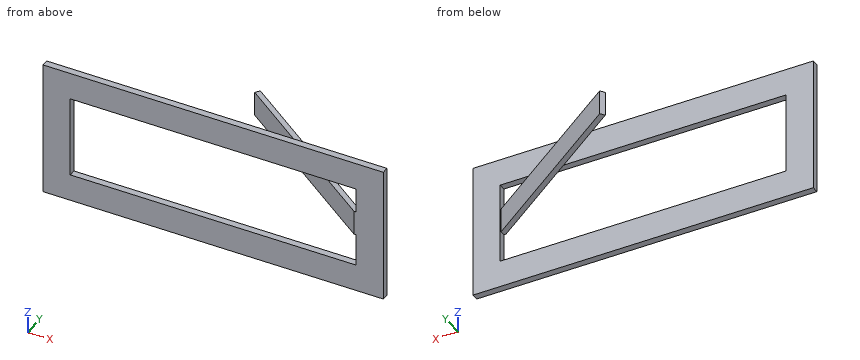
```python
from build123d import *

# Parameters (mm, degrees)
SKETCH1_W           = 20
SKETCH1_H           = 60
BOSS_EXTRUDE2_DEPTH = 10
BOSS_EXTRUDE3_DEPTH = 36
SKETCH3_W           = 140
SKETCH3_H           = 140
CUT_EXTRUDE1_DEPTH  = 18
SKETCH4_W           = 8.585490735
SKETCH4_H           = 18
CUT_EXTRUDE3_DEPTH  = 46
SKETCH5_W           = 250
SKETCH5_H           = 5
CUT_EXTRUDE4_DEPTH  = 137


with BuildPart() as part:
    # Sketch1 → Boss-Extrude2 (new body)
    with BuildSketch(Plane(origin=(0, 0, 0), x_dir=(1, 0, 0), z_dir=(0, 1, 0))):
        Polygon((166.222222222, 60), (146.222222222, 60), (-63.777777778, 60), (-83.777777778, 60), (-83.777777778, 80), (166.222222222, 80), align=None)
        with Locations((156.222222222, 30)):
            Rectangle(SKETCH1_W, SKETCH1_H)
        Polygon((166.222222222, 0), (146.222222222, 0), (-63.777777778, 0), (-83.777777778, 0), (-83.777777778, -20), (166.222222222, -20), align=None)
        with Locations((-73.777777778, 30)):
            Rectangle(SKETCH1_W, SKETCH1_H)
    extrude(amount=BOSS_EXTRUDE2_DEPTH)

    # Sketch2 → Boss-Extrude3 (add)
    with BuildSketch(Plane.XY):
        Polygon((155.307951765, 2.266232377), (27.198414629, 93.999150061), (24.869662654, 90.746933242), (148.437318839, 2.266232377), align=None)
    extrude(amount=-BOSS_EXTRUDE3_DEPTH)

    # Sketch3 → Cut-Extrude1 (cut)
    with BuildSketch(Plane.XY):
        with Locations((82.194738609, 80)):
            Rectangle(SKETCH3_W, SKETCH3_H)
    extrude(amount=-CUT_EXTRUDE1_DEPTH, mode=Mode.SUBTRACT)

    # Sketch4 → Cut-Extrude3 (cut)
    with BuildSketch(Plane(origin=(0, 10, 0), x_dir=(1, 0, 0), z_dir=(0, 1, 0))):
        with Locations((141.929476855, 9)):
            Rectangle(SKETCH4_W, SKETCH4_H)
    extrude(amount=-CUT_EXTRUDE3_DEPTH, mode=Mode.SUBTRACT)

    # Sketch5 → Cut-Extrude4 (cut)
    with BuildSketch(Plane.XY.offset(20)):
        with Locations((41.222222222, 2.5)):
            Rectangle(SKETCH5_W, SKETCH5_H)
    extrude(amount=-CUT_EXTRUDE4_DEPTH, mode=Mode.SUBTRACT)


solid = part.part
```
The model under review builds one solid part; all positions refer to its coordinate system, in mm. Give positions to 0.01 mm unless a question says otherwise; leave off trailing zeros. Write each loop counter-clockwise with the first axis right and the second up, starting at its lowest first coordinate (ties: lowest second). Pieces come first, ordered by that corner, then holes.
(1) Consider section B-B, the plane x = 8.5. Give the boundary of the cut face in (y, z).
(2) Consider section C-C, the plane x = 140. Give the boundary of the cut face in (y, z).
(3) Consider section A-A, the plane z = -8.5. Give the boundary of the cut face in (x, y).
(4) Consider section D-D, the plane z = -28. Give the boundary of the cut face in (x, y), and give its area (3 significant figures).
(5) To check wall thickness, follow L1, parallel to Y at x = 36.5, z = -64; L2, parallel to Y at x = 32.5, z = -22.5; L3, parallel to X at y = 62, z = -33.5. State the ranges of each line that lie inside material, in increasing order.
(6) For P1, Ø2, axis at x = 113, z = -18, coming from the -Y side; P2, Ø4, axis at x = -30, z = -61, coming from the +Y side; P3, Ø6, axis at x = -54, z = -54.5, coming from the -Y side, all flat-tipped, find the tip position at first contact; note any pin that passes through.
Returned:
1. outline: (5, -80) - (10, -80) - (10, -60) - (5, -60) - close; (5, 0) - (10, 0) - (10, 20) - (5, 20) - close
2. outline: (5, -80) - (10, -80) - (10, -60) - (5, -60) - close; (5, 0) - (10, 0) - (10, 20) - (5, 20) - close; (8.31, -36) - (13.23, -36) - (13.23, -18) - (8.31, -18) - close
3. outline: (-83.78, 5) - (-63.78, 5) - (-63.78, 10) - (-83.78, 10) - close; (146.22, 5) - (166.22, 5) - (166.22, 10) - (146.22, 10) - close
4. outline: (-83.78, 5) - (-63.78, 5) - (-63.78, 10) - (-83.78, 10) - close; (24.87, 90.75) - (144.62, 5) - (166.22, 5) - (166.22, 10) - (146.22, 10) - (146.22, 8.77) - (27.2, 94) - close
4. area: 790 mm2
5. L1: y = 5 to 10
5. L2: y = 85.28 to 90.2
5. L3: x = 65.02 to 71.89
6. P1: stops at y = 26.93
6. P2: stops at y = 10
6. P3: passes through
